Here's how the part is built. I have some questions about the finished solid (model axes, mm). Round coordinates to 2 decimals unless told otherwise and drop trailing zeros. Order: outer loops, then holes, each group sorted by start corner. A loop starts at its lowest first (then second) coordinate and runs counter-clockwise, first axis right, second up. Notation, with made-up numbers: (-3.75, 7) -> (15.25, 7) arc R18 ccw to (15.25, 36) -> close; hole circle Ø4 at (84, -6). An arc over 180 degrees is marked (long way). One line per item, written item: value.
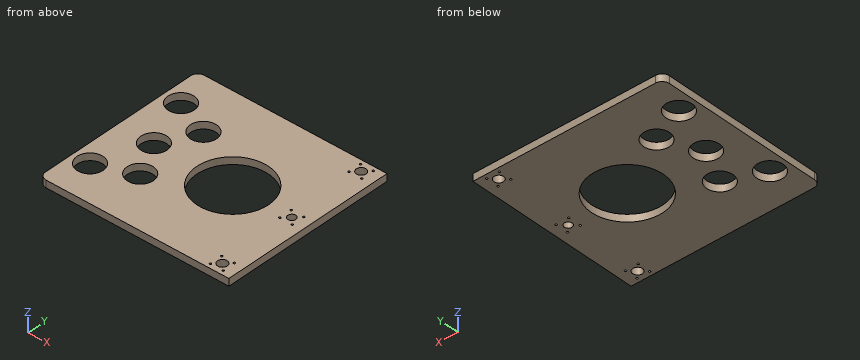
```python
from build123d import *

# Parameters (mm, degrees)
SKETCH_1_W          = 530
SKETCH_1_H          = 490
SKETCH_1_R          = 36.5
SKETCH_1_R_2        = 11
SKETCH_1_R_3        = 2.75
SKETCH_1_R_4        = 13.5
EXTRUDE_1_DEPTH     = 20
FILLET_1_R          = 20
SKETCH_2_R          = 100
CUT_EXTRUDE_1_DEPTH = 496.302937605


with BuildPart() as part:
    # Sketch 1 → Extrude 1 (new body)
    with BuildSketch(Plane.XY):
        with Locations((165, 0)):
            Rectangle(SKETCH_1_W, SKETCH_1_H)
        Circle(SKETCH_1_R, mode=Mode.SUBTRACT)
        with Locations((50, 97.979589711)):
            Circle(SKETCH_1_R, mode=Mode.SUBTRACT)
        with Locations((50, -97.979589711)):
            Circle(SKETCH_1_R, mode=Mode.SUBTRACT)
        with Locations((-51.249933939, 140.973204089)):
            Circle(SKETCH_1_R, mode=Mode.SUBTRACT)
        with Locations((-51.249933939, -140.973204089)):
            Circle(SKETCH_1_R, mode=Mode.SUBTRACT)
        with Locations((385, 0)):
            Circle(SKETCH_1_R_2, mode=Mode.SUBTRACT)
        with Locations((367.32233047, 17.67766953)):
            Circle(SKETCH_1_R_3, mode=Mode.SUBTRACT)
        with Locations((402.67766953, 17.67766953)):
            Circle(SKETCH_1_R_3, mode=Mode.SUBTRACT)
        with Locations((367.32233047, -17.67766953)):
            Circle(SKETCH_1_R_3, mode=Mode.SUBTRACT)
        with Locations((402.67766953, -17.67766953)):
            Circle(SKETCH_1_R_3, mode=Mode.SUBTRACT)
        with Locations((385, 215)):
            Circle(SKETCH_1_R_4, mode=Mode.SUBTRACT)
        with Locations((367.32233047, 197.32233047)):
            Circle(SKETCH_1_R_3, mode=Mode.SUBTRACT)
        with Locations((402.67766953, 197.32233047)):
            Circle(SKETCH_1_R_3, mode=Mode.SUBTRACT)
        with Locations((402.67766953, 232.67766953)):
            Circle(SKETCH_1_R_3, mode=Mode.SUBTRACT)
        with Locations((367.32233047, 232.67766953)):
            Circle(SKETCH_1_R_3, mode=Mode.SUBTRACT)
        with Locations((367.32233047, -232.67766953)):
            Circle(SKETCH_1_R_3, mode=Mode.SUBTRACT)
        with Locations((402.67766953, -232.67766953)):
            Circle(SKETCH_1_R_3, mode=Mode.SUBTRACT)
        with Locations((402.67766953, -197.32233047)):
            Circle(SKETCH_1_R_3, mode=Mode.SUBTRACT)
        with Locations((367.32233047, -197.32233047)):
            Circle(SKETCH_1_R_3, mode=Mode.SUBTRACT)
        with Locations((385, -215)):
            Circle(SKETCH_1_R_4, mode=Mode.SUBTRACT)
    extrude(amount=EXTRUDE_1_DEPTH)

    # Fillet 1
    fillet_1_edges = [part.edges().sort_by_distance(p)[0] for p in [
        (-100, -245, 10),
        (-100, 245, 10),
    ]]
    fillet(fillet_1_edges, radius=FILLET_1_R)

    # Sketch 2 → Cut-Extrude 1 (cut, through all)
    with BuildSketch(Plane.XY.offset(20)):
        with Locations((220, 0)):
            Circle(SKETCH_2_R)
    extrude(amount=-CUT_EXTRUDE_1_DEPTH, mode=Mode.SUBTRACT)


solid = part.part
```
Q1. I want a section at A-A on y = 0. Write out the boundary of the cut face in (x, z).
Answers:
outline: (-100, 0) -> (-36.5, 0) -> (-36.5, 20) -> (-100, 20) -> close; (36.5, 0) -> (120, 0) -> (120, 20) -> (36.5, 20) -> close; (320, 0) -> (374, 0) -> (374, 20) -> (320, 20) -> close; (396, 0) -> (430, 0) -> (430, 20) -> (396, 20) -> close
Q2. I want a section at D-D on x = 385. Write out the boundary of the cut face in (y, z), then the cut area to 3 significant figures.
Answers:
outline: (-245, 0) -> (-228.5, 0) -> (-228.5, 20) -> (-245, 20) -> close; (-201.5, 0) -> (-11, 0) -> (-11, 20) -> (-201.5, 20) -> close; (11, 0) -> (201.5, 0) -> (201.5, 20) -> (11, 20) -> close; (228.5, 0) -> (245, 0) -> (245, 20) -> (228.5, 20) -> close
area: 8,280 mm2
Q3. For P1, Ø6.5, axis at x = 402.68, y = -17.68, coming from the +Z side, with a flat end and sliding along its axis, tell me the tip position at first contact or that it passes through.
Answers:
P1: z = 20
Q4. I need wall thicknesses on line 1 along X through (y, z) = (-28.5, 7); line 2 along Y through (x, z) = (225, 8.5); line 3 along X through (y, z) = (-195, 1.75). Which ranges of each line are inside material? Lowest first, please.
Answers:
line 1: -100 to -22.8, 22.8 to 124.15, 315.85 to 430
line 2: -245 to -99.87, 99.87 to 245
line 3: -100 to 365.85, 368.8 to 401.2, 404.15 to 430
Q5. I want a section at B-B on x = 220. Write out the boundary of the cut face in (y, z).
Answers:
outline: (-245, 0) -> (-100, 0) -> (-100, 20) -> (-245, 20) -> close; (100, 0) -> (245, 0) -> (245, 20) -> (100, 20) -> close
Q6. I want a section at C-C on y = -215. Write out the boundary of the cut face in (x, z).
Answers:
outline: (-100, 0) -> (371.5, 0) -> (371.5, 20) -> (-100, 20) -> close; (398.5, 0) -> (430, 0) -> (430, 20) -> (398.5, 20) -> close
